from build123d import *

# Parameters (mm, degrees)
SKETCH2_R           = 30
SKETCH2_R_2         = 25
BOSS_EXTRUDE1_DEPTH = 15
BOSS_EXTRUDE2_DEPTH = 20
SKETCH5_R           = 10
SKETCH5_R_2         = 15
CUT_EXTRUDE2_DEPTH  = 40


with BuildPart() as part:
    # Sketch2 → Boss-Extrude1 (new body, symmetric)
    with BuildSketch(Plane.XY):
        with BuildLine():
            Line((183.28793901, 60), (21.361321264, 109.891650199))
            ThreePointArc((21.361321264, 109.891650199), (34.112595949, 100.848686279), (39, 86))
            ThreePointArc((39, 86), (16.637488364, 61.139516193), (-10.44349241, 80.754461058))
            ThreePointArc((-10.44349241, 80.754461058), (-10.481072196, 47.848151082), (-24.085330203, 17.885660989))
            ThreePointArc((-24.085330203, 17.885660989), (9.419131964, 28.482976548), (30, 0))
            ThreePointArc((30, 0), (27.440845468, -12.124355653), (20.2, -22.180171325))
            ThreePointArc((20.2, -22.180171325), (106.532601106, 8.971535214), (189.628727834, -30))
            Line((189.628727834, -30), (270, -30))
            Line((270, -30), (270, -3))
            Line((270, -3), (183.28793901, 60))
        make_face()
        Circle(SKETCH2_R)
        with Locations((14, 86)):
            Circle(SKETCH2_R_2)
    extrude(amount=BOSS_EXTRUDE1_DEPTH, both=True)

    # Sketch4 → Boss-Extrude2 (add, symmetric)
    with BuildSketch(Plane.XY):
        with BuildLine():
            Line((189.628727834, -30), (270, -30))
            Line((270, -30), (270, -3))
            Line((270, -3), (183.28793901, 60))
            Line((183.28793901, 60), (21.361321264, 109.891650199))
            ThreePointArc((21.361321264, 109.891650199), (-2.887690503, 104.433825145), (-10.44349241, 80.754461058))
            ThreePointArc((-10.44349241, 80.754461058), (-10.481072196, 47.848151082), (-24.085330203, 17.885660989))
            ThreePointArc((-24.085330203, 17.885660989), (-20.126889413, -22.246535068), (20.2, -22.180171325))
            ThreePointArc((20.2, -22.180171325), (106.532601106, 8.971535214), (189.628727834, -30))
        make_face()
        with BuildLine():
            Line((193.090377844, -22), (262, -22))
            Line((262, -22), (262, -7.076203596))
            Line((262, -7.076203596), (179.661480345, 52.746232627))
            Line((179.661480345, 52.746232627), (19.00569846, 102.246322136))
            ThreePointArc((19.00569846, 102.246322136), (2.516370458, 98.535001099), (-2.621574839, 82.43303352))
            ThreePointArc((-2.621574839, 82.43303352), (-2.663008962, 46.151717392), (-17.662575482, 13.116151392))
            ThreePointArc((-17.662575482, 13.116151392), (-14.759718903, -16.314125717), (14.813333333, -16.265458972))
            ThreePointArc((14.813333333, -16.265458972), (105.1151782, 17.032975134), (193.090377844, -22))
        make_face(mode=Mode.SUBTRACT)
    extrude(amount=BOSS_EXTRUDE2_DEPTH, both=True)

    # Sketch5 → Cut-Extrude2 (cut)
    with BuildSketch(Plane.XY.offset(15)):
        with Locations((14, 86)):
            Circle(SKETCH5_R)
        Circle(SKETCH5_R_2)
    extrude(amount=-CUT_EXTRUDE2_DEPTH, mode=Mode.SUBTRACT)


solid = part.part
Here's how the part is built. I have some questions about the finished solid (model axes, mm). A direction names the side the tool comes from. Coordinates: 2 decimals unless noted, no trailing zeros. Order: outer loops, then holes, each group sorted by start corner. A loop starts at its lowest first (then second) coordinate and runs counter-clockwise, first axis right, second up.
Item 1: For P1, Ø12, axis at y = 39.5, z = -8.5, coming from the +X side; P2, Ø2, axis at y = 23.5, z = 2.5, coming from the +X side; P3, Ø1.5, axis at y = -12, z = -18, coming from the -X side; P4, Ø18, axis at x = 0, y = 0, coming from the +Z side, each with a flat end and sliding along its axis, tell me the tip position at first contact or that it passes through.
Result sheet:
P1: stops at x = 219.76
P2: stops at x = 234.9
P3: stops at x = -27.81
P4: passes through
Item 2: I need wall thicknesses on line 1 (X direction, y = -7.5, z = -16); line 2 (X direction, y = -2, z = 10.5); line 3 (Z direction, x = 78.5, y = 20.5). Which ranges of each line are inside material? Lowest first, please.
Result sheet:
line 1: x = -29.05 to -20.68, 25.55 to 40.1, 161.9 to 176.45, 262 to 270
line 2: x = -29.93 to -14.87, 14.87 to 50.6, 151.4 to 268.62
line 3: z = -15 to 15
Item 3: If we section it at C-C on z = -0.5: List the corners of the cut face in (x, y) for me, plus the area to 3 significant figures.
Result sheet:
outline: (-24.09, 17.89) arc R30 ccw to (20.2, -22.18) arc R120 cw to (189.63, -30) - (270, -30) - (270, -3) - (183.29, 60) - (21.36, 109.89) arc R25 ccw to (-10.44, 80.75) arc R78 cw to start; hole circle Ø30 at (0, 0); hole circle Ø20 at (14, 86)
area: 23,100 mm2
Item 4: If we mould it in two halves opening along X, with no side actions, what happens to faces 4 (the face through (-2.556, 46.652, -17.465)), 5 (the face through (270, -17, 0)), 6 (the face through (229, -30, 0))? For each: +X half, -X half, draft (parallel to the pull), parting line (faces both ways), or undercut.
Result sheet:
face 4: undercut
face 5: +X half
face 6: draft
Item 5: For faces 1 (the face through (103.458, 84.597, 0.28)), 2 (the face through (2.7, 98.7, -17.5)), 3 (the face through (221.407, 22.416, 17.535)), which set-ups out of +Z, -Z, +X, -X, +Y, -Y let a thin tool reach every point of the face, with its end or its side?
Result sheet:
face 1: +Z, -Z, +X, +Y
face 2: -Z
face 3: +Z
Item 6: If we section it at A-A on y = 86: List the corners of the cut face in (x, z) for me, plus the area to 3 significant figures.
Result sheet:
outline: (-11, -20) - (-3, -20) - (-3, -15) - (4, -15) - (4, 15) - (-3, 15) - (-3, 20) - (-11, 20) - close; (24, -15) - (71.73, -15) - (71.73, -20) - (98.9, -20) - (98.9, 20) - (71.73, 20) - (71.73, 15) - (24, 15) - close
area: 3,050 mm2
Item 7: If we section it at D-D on x = 123: List the corners of the cut face in (y, z) for me, plus the area to 3 significant figures.
Result sheet:
outline: (7.07, -20) - (15.19, -20) - (15.19, -15) - (70.2, -15) - (70.2, -20) - (78.58, -20) - (78.58, 20) - (70.2, 20) - (70.2, 15) - (15.19, 15) - (15.19, 20) - (7.07, 20) - close
area: 2,310 mm2
Item 8: If we section it at B-B on y = 0: List the corners of the cut face in (x, z) for me, plus the area to 3 significant figures.
Result sheet:
outline: (-30, -20) - (-22, -20) - (-22, -15) - (-15, -15) - (-15, 15) - (-22, 15) - (-22, 20) - (-30, 20) - close; (15, -15) - (37.09, -15) - (37.09, -20) - (55.16, -20) - (55.16, 20) - (37.09, 20) - (37.09, 15) - (15, 15) - close; (146.84, -20) - (164.91, -20) - (164.91, -15) - (252.26, -15) - (252.26, -20) - (265.87, -20) - (265.87, 20) - (252.26, 20) - (252.26, 15) - (164.91, 15) - (164.91, 20) - (146.84, 20) - close
area: 5,800 mm2
